Design review of the part built by this model. Coordinates are the model's own, in mm. Face numbers are marked on the shaded views. A direction names the side the tool comes from. Coordinates: 2 decimals unless noted, no trailing zeros. Write each loop counter-clockwise with the first axis right and the second up, starting at its lowest first coordinate (ties: lowest second). Pieces come first, ordered by that corner, then holes.
Q1. Mouldability with a two-part tool opening along X and no side actions: class the marked faces 3, 4 and 5 as pulls with the +X half, pulls with the -X half, needs draft (parallel to the pull), parting line crosses it, or undercut.
Q2. Take a section at D-D (x = -44). Give the boundary of the cut face in (y, z) (3 decimals).
Q3. Take a section at A-A (z = 9.5). Give the boundary of the cut face in (x, y).
Q4. Machinability: for the marked faces 1 and 2, which of the approach directions +Z, -Z, +X, -X, +Y, -Y give a long, thin tool a straight path to every point of the face, cutting with its end or side? Answer none if there is none.
Q5. For probe 1 along Z at (x, y) = (-38, 41.5); probe 2 along X at (y, z) = (-12, 6.25); probe 3 along X at (y, z) = (63.5, 12.5), list the stretches that pass through material, from the lowest coordinate up.
Q6. Take a section at C-C (y = 84.5). Give the boundary of the cut face in (x, z), and give its area (3 significant figures).
Q7. Take a section at B-B (x = -2.5). Give the boundary of the cut face in (y, z) (3 decimals), and give its area (3 significant figures).
Q8. Insertion check: pin 1 (2 mm diameter, centred on x = -13, y = 36, fed in from +Z); pin 2 (8 mm diameter, centred on y = 43, z = 5, fed in from -X); pin 3 (1.8 mm diameter, centred on x = 10.5, y = 55, fed in from +Z) (3 decimals); pin 4 (16.5 mm diameter, centred on x = -38, y = -17.5, fed in from +Z). Each pin has a flat end and moves straight along its axis. Give the tip position at first contact, or say it passes through.
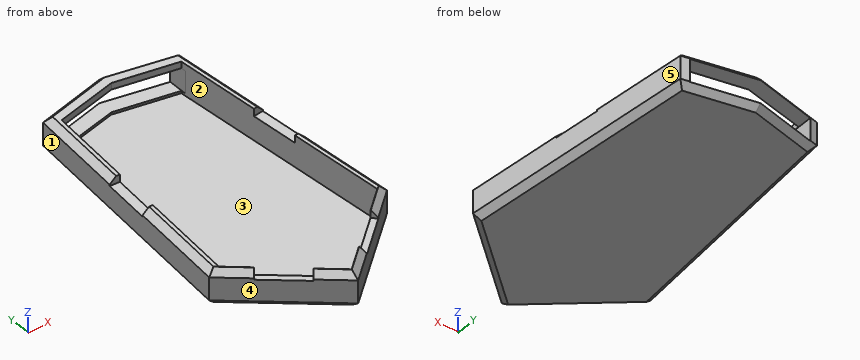
```python
from build123d import *

# Parameters (mm, degrees)
BOSS_EXTRUDE1_DEPTH = 15
BOSS_EXTRUDE2_DEPTH = 1.5
SKETCH4_W           = 51.62387155
SKETCH4_H           = 9.672418812
CUT_EXTRUDE2_DEPTH  = 144.5
SKETCH9_W           = 20
SKETCH9_H           = 3.175
CUT_EXTRUDE3_DEPTH  = 5.5
SKETCH6_W           = 3.175
SKETCH6_H           = 20
CUT_EXTRUDE4_DEPTH  = 5.5
SKETCH8_W           = 20
SKETCH8_H           = 3.175
CUT_EXTRUDE5_DEPTH  = 5.5
SKETCH7_W           = 3.175
SKETCH7_H           = 20
CUT_EXTRUDE6_DEPTH  = 5.5
CHAMFER1_SIZE       = 2.6


with BuildPart() as part:
    # Sketch1 → Boss-Extrude1 (new body)
    with BuildSketch(Plane.XY):
        Polygon((-59.040836406, -0.235043033), (-20.940836406, -32.613894155), (17.159163594, -0.235043033), (8.348043807, 100.476516972), (-20.940836406, 106.96970539), (-50.22971662, 100.476516972), align=None)
        Polygon((-46.574564783, 95.01395338), (-20.940836406, 100.476516972), (4.69289197, 95.01395338), (13.026099369, -0.235043033), (-20.940836406, -29.10145659), (-54.907772181, -0.235043033), align=None, mode=Mode.SUBTRACT)
    extrude(amount=BOSS_EXTRUDE1_DEPTH)

    # Sketch1<6> → Boss-Extrude2 (add)
    with BuildSketch(Plane.XY):
        Polygon((-54.907772181, -0.235043033), (-46.574564783, 95.01395338), (-20.940836406, 100.476516972), (4.69289197, 95.01395338), (13.026099369, -0.235043033), (-20.940836406, -29.10145659), align=None)
    extrude(amount=BOSS_EXTRUDE2_DEPTH)

    # Sketch4 → Cut-Extrude2 (cut)
    with BuildSketch(Plane(origin=(0, 0, 0), x_dir=(1, 0, 0), z_dir=(0, 1, 0))):
        with Locations((-20.940836406, -7.336209406)):
            Rectangle(SKETCH4_W, SKETCH4_H)
    extrude(amount=CUT_EXTRUDE2_DEPTH, mode=Mode.SUBTRACT)

    # Sketch9 → Cut-Extrude3 (cut)
    with BuildSketch(Plane(origin=(7.31178106, -8.603728938, 0), x_dir=(0.7619999999999999, 0.6475770224459791, 0), z_dir=(0.6475770224459791, -0.7619999999999999, 0))):
        with Locations((-12.076925809, 13.4125)):
            Rectangle(SKETCH9_W, SKETCH9_H)
    extrude(amount=-CUT_EXTRUDE3_DEPTH, mode=Mode.SUBTRACT)

    # Sketch6 → Cut-Extrude4 (cut)
    with BuildSketch(Plane(origin=(17.008413071, 1.488043328, 0), x_dir=(0, 0, -1), z_dir=(0.9961946980917459, 0.08715574274765506, 0))):
        with Locations((-13.4125, 48.820331729)):
            Rectangle(SKETCH6_W, SKETCH6_H)
    extrude(amount=-CUT_EXTRUDE4_DEPTH, mode=Mode.SUBTRACT)

    # Sketch8 → Cut-Extrude5 (cut)
    with BuildSketch(Plane(origin=(-24.875111844, -29.270394977, 0), x_dir=(0.7620000000000001, -0.6475770224459789, 0), z_dir=(-0.6475770224459789, -0.7620000000000001, 0))):
        with Locations((-19.836908874, 13.4125)):
            Rectangle(SKETCH8_W, SKETCH8_H)
    extrude(amount=-CUT_EXTRUDE5_DEPTH, mode=Mode.SUBTRACT)

    # Sketch7 → Cut-Extrude6 (cut)
    with BuildSketch(Plane(origin=(-58.571947524, 5.124381409, 0), x_dir=(0, 0, 1), z_dir=(-0.996194698091746, 0.0871557427476544, 0))):
        with Locations((13.4125, 45.170103428)):
            Rectangle(SKETCH7_W, SKETCH7_H)
    extrude(amount=-CUT_EXTRUDE6_DEPTH, mode=Mode.SUBTRACT)

    # Chamfer1
    # the kernel refuses this chamfer: 2.6 mm, written as the material it takes off along each edge
    with BuildSketch(Plane(origin=(-14.412954441, 108.41690198, 0), x_dir=(0.2163577817803448, -0.9759268861100734, -0.027495876610586355), z_dir=(-0.976296007119934, -0.21643961393810024, 0)), Plane(origin=(-14.412954441, 108.41690198, 15), x_dir=(-0.0059511969184851, 0.026844114547178517, -0.9996219169112966), z_dir=(-0.976296007119934, -0.21643961393810024, 0)), Plane(origin=(14.875925773, 99.029320382, 15), x_dir=(0.0059511969184853734, 0.026844114547178898, -0.9996219169112966), z_dir=(-0.9762960071199325, 0.2164396139381068, 0)), Plane(origin=(14.875925773, 99.029320382, 0), x_dir=(-0.21635778178035134, -0.9759268861100718, -0.027495876610586386), z_dir=(-0.9762960071199325, 0.2164396139381068, 0))) as chamfer1_piece_1:
        Polygon((CHAMFER1_SIZE * 0.999621916911, CHAMFER1_SIZE * 0.0274958766106), (-CHAMFER1_SIZE * 0.0274958766106, CHAMFER1_SIZE * 0.999621916911), (0, 0), align=None)
    extrude(amount=43.372751537, mode=Mode.SUBTRACT)
    with BuildSketch(Plane(origin=(-49.646960573, 107.137449062, 0), x_dir=(0.9958180537233415, -0.0871227906352381, -0.02749587661058639), z_dir=(-0.08715574274765436, -0.9961946980917459, 0)), Plane(origin=(17.74191964, -6.895975123, 0), x_dir=(-0.9958180537233413, -0.08712279063523876, -0.027495876610586372), z_dir=(-0.08715574274765503, 0.9961946980917459, 0))) as chamfer1_piece_2:
        Polygon((CHAMFER1_SIZE * 0.999621916911, CHAMFER1_SIZE * 0.0274958766106), (-CHAMFER1_SIZE * 0.0274958766106, CHAMFER1_SIZE * 0.999621916911), (0, 0), align=None)
    extrude(amount=114.46901334, mode=Mode.SUBTRACT)
    with BuildSketch(Plane(origin=(-64.135854742, 4.094900279, 0), x_dir=(-0.017805697905026136, -0.02095185797726749, 0.9996219169112966), z_dir=(0.762, -0.6475770224459791, 0))) as chamfer1_piece_3:
        Polygon((CHAMFER1_SIZE * 0.999621916911, -CHAMFER1_SIZE * 0.0274958766106), (-CHAMFER1_SIZE * 0.0274958766106, -CHAMFER1_SIZE * 0.999621916911), (0, 0), align=None)
    extrude(amount=63.372751537, mode=Mode.SUBTRACT)
    with BuildSketch(Plane(origin=(-26.035854742, -36.943837466, 0), x_dir=(-0.6473321845251594, 0.761711900686408, -0.027495876610586337), z_dir=(0.762, 0.6475770224459791, 0))) as chamfer1_piece_4:
        Polygon((CHAMFER1_SIZE * 0.999621916911, CHAMFER1_SIZE * 0.0274958766106), (-CHAMFER1_SIZE * 0.0274958766106, CHAMFER1_SIZE * 0.999621916911), (0, 0), align=None)
    extrude(amount=63.372751537, mode=Mode.SUBTRACT)
    with BuildSketch(Plane(origin=(-26.035854742, -36.943837466, 15), x_dir=(0.017805697905026178, -0.02095185797726754, -0.9996219169112966), z_dir=(0.762, 0.6475770224459791, 0)), Plane(origin=(-37.465854742, -18.570295507, 15), x_dir=(-0.017805697905026636, -0.020951857977268076, -0.9996219169112966), z_dir=(0.762, -0.6475770224459791, 0)), Plane(origin=(-64.135854742, 4.094900279, 15), x_dir=(-0.017805697905026147, -0.0209518579772675, -0.9996219169112966), z_dir=(0.762, -0.6475770224459791, 0)), Plane(origin=(0.634145258, -14.278641681, 15), x_dir=(0.017805697905025515, -0.020951857977266758, -0.9996219169112966), z_dir=(0.762, 0.6475770224459791, 0))) as chamfer1_piece_5:
        Polygon((CHAMFER1_SIZE * 0.999621916911, CHAMFER1_SIZE * 0.0274958766106), (-CHAMFER1_SIZE * 0.0274958766106, CHAMFER1_SIZE * 0.999621916911), (0, 0), align=None)
    extrude(amount=28.372751537, mode=Mode.SUBTRACT)
    with BuildSketch(Plane(origin=(-54.923914991, 46.821584065, 15), x_dir=(0.9958180537233415, -0.0871227906352381, 0.027495876610586705), z_dir=(-0.08715574274765436, -0.9961946980917459, 0))) as chamfer1_piece_6:
        Polygon((CHAMFER1_SIZE * 0.999621916911, -CHAMFER1_SIZE * 0.0274958766106), (-CHAMFER1_SIZE * 0.0274958766106, -CHAMFER1_SIZE * 0.999621916911), (0, 0), align=None)
    extrude(amount=53.922751537, mode=Mode.SUBTRACT)
    with BuildSketch(Plane(origin=(-49.646960573, 107.137449062, 15), x_dir=(-0.02739124649885124, 0.002396423548493534, -0.9996219169112966), z_dir=(-0.08715574274765436, -0.9961946980917459, 0)), Plane(origin=(12.464639417, 53.423613846, 15), x_dir=(0.027391246498851204, 0.0023964235484935496, -0.9996219169112966), z_dir=(-0.08715574274765503, 0.9961946980917459, 0))) as chamfer1_piece_7:
        Polygon((CHAMFER1_SIZE * 0.999621916911, CHAMFER1_SIZE * 0.0274958766106), (-CHAMFER1_SIZE * 0.0274958766106, CHAMFER1_SIZE * 0.999621916911), (0, 0), align=None)
    extrude(amount=53.91901334, mode=Mode.SUBTRACT)
    with BuildSketch(Plane(origin=(17.74191964, -6.895975123, 15), x_dir=(0.027391246498850576, 0.0023964235484934945, -0.9996219169112966), z_dir=(-0.08715574274765503, 0.9961946980917459, 0))) as chamfer1_piece_8:
        Polygon((CHAMFER1_SIZE * 0.999621916911, CHAMFER1_SIZE * 0.0274958766106), (-CHAMFER1_SIZE * 0.0274958766106, CHAMFER1_SIZE * 0.999621916911), (0, 0), align=None)
    extrude(amount=53.922751537, mode=Mode.SUBTRACT)


solid = part.part
```
Response:
1. face 3: undercut
1. face 4: pulls with the -X half
1. face 5: pulls with the +X half
2. outline: (-13.017, 2.6) - (-9.605, 0) - (99.194, 0) - (101.755, 2.5) - (95.563, 2.5) - (95.563, 1.5) - (-9.505, 1.5) - (-9.505, 11.825) - (-13.017, 11.825) - close; (95.563, 12.172) - (101.858, 12.172) - (101.858, 12.4) - (99.194, 15) - (95.563, 15) - close
3. outline: (-59.04, -0.24) - (-20.94, -32.61) - (17.16, -0.24) - (8.35, 100.48) - (4.87, 101.25) - (4.87, 92.98) - (13.03, -0.24) - (-20.94, -29.1) - (-54.91, -0.24) - (-46.75, 92.98) - (-46.75, 101.25) - (-50.23, 100.48) - close
4. face 1: +Z, -Z, -X, +Y
4. face 2: +Z
5. probe 1: z = 0 to 1.5
5. probe 2: x = -45.2 to -41.06, -0.82 to 3.32
5. probe 3: x = -53.36 to -49.33, 7.45 to 11.48
6. outline: (-51.63, 2.6) - (-49.02, 0) - (7.14, 0) - (9.75, 2.6) - (9.75, 12.4) - (7.14, 15) - (5.61, 15) - (5.61, 1.5) - (-47.49, 1.5) - (-47.49, 15) - (-49.02, 15) - (-51.63, 12.4) - close
6. area: 190 mm2
7. outline: (-16.942, 2.6) - (-13.53, 0) - (100.218, 0) - (102.779, 2.5) - (96.547, 2.5) - (96.547, 1.5) - (-13.43, 1.5) - (-13.43, 11.825) - (-16.942, 11.825) - close; (96.547, 12.172) - (102.881, 12.172) - (102.881, 12.4) - (100.218, 15) - (96.547, 15) - close
7. area: 229 mm2
8. pin 1: stops at z = 1.5
8. pin 2: stops at x = -55.61
8. pin 3: stops at z = 11.825
8. pin 4: stops at z = 15
